Input: part model. Units: mm. Frame: model coordinates. A direction names the side the tool comes from. Coordinates: 2 decimals unless noted, no trailing zeros. Write each loop counter-clockwise with the first axis right and the second up, starting at its lowest first coordinate (ties: lowest second). Pieces come first, ordered by that corner, then holes. Notation, with made-up numbers: (62, -2) - (85, -2) arc R14 cw to (85, 2) - close; hole circle Ø10 at (85.25, -9). An arc over 180 degrees is marked (long way). Use a Markdown table: item, result. Add a question column.
Q1. Mould query, pull axis X, two halves, no side actions, for faces 1 (the face through (-5.568, -4.93, -17.725)), 2 (the face through (4, -10, 11)), 3 (the face through (-8.099, -15.21, 7.597)), 4 (the face through (-20.331, -5, 2)). Classes: released by +X, released by -X, zero draft, split by the parting line, or undercut.
Q2. Set-up query: faces 5 (the face through (-17.32, -19.86, 2.8)), 6 (the face through (9.669, -5, 2)). Return all of +Z, -Z, +X, -X, +Y, -Y with unobstructed straight access to the full face (end or side cutting, diameter ignored); none if empty.
Q3. Section query A-A (z = -2.5). Return the cut outline in (x, y).
Q4. Material intervals for probe 1 along X at (y, z) = (-23.25, 7); probe 2 along Y at (x, z) = (-16.5, 7); probe 3 along X at (y, z) = (-20, 5), sorted ascending. Write a range as from..to.
Q5. Section query D-D (x = -5). Return the cut outline in (y, z), then the cut area to 3 significant figures.
Q6. Section query C-C (y = -8.5). Give the number of separate pieces and of enclosed holes in the cut face, then the cut area to 3 significant figures.
Q7. Section query B-B (x = -1). Return the cut outline in (y, z), then the cut area to 3 significant figures.
Q8. Pin query (flat end, axial travel): P1, Ø6, axis at x = -12, y = -21, coming from the +Z side; P2, Ø1, axis at x = -2.5, z = 6.5, coming from the +Y side; P3, Ø6, axis at y = -25, z = 13.5, coming from the +X side; P4, Ø12, axis at y = -25, z = -5, coming from the +X side. Return the tip coordinate at first contact, or that it passes through.
from build123d import *

# Parameters (mm, degrees)
F0_R     = 12
F1_DEPTH = 10
F2_DEPTH = 30
F3_D     = 12
F3_DEPTH = 50
F3_TIP   = 3.6051637142


with BuildPart() as f1:
    # F0 (on Front) → F1 (new body)
    with BuildSketch(Plane.XZ):
        with BuildLine():
            Line((9.6692045312, -3.2938710881), (9.6692045312, 7.8416576376))
            ThreePointArc((9.6692045312, 7.8416576376), (8.7102254474, 9.9452511488), (7.4580991057, 11.8886826932))
            ThreePointArc((7.4580991057, 11.8886826932), (4.3919227725, 11.9966115161), (4.2839939496, 15.0627878494))
            ThreePointArc((4.2839939496, 15.0627878494), (0.792139449, 17.055965795), (-3.0863641887, 18.1156901498))
            ThreePointArc((-3.0863641887, 18.1156901498), (-5.3307954688, 16.0238932748), (-7.575226749, 18.1156901498))
            ThreePointArc((-7.575226749, 18.1156901498), (-11.4537303867, 17.055965795), (-14.9455848872, 15.0627878494))
            ThreePointArc((-14.9455848872, 15.0627878494), (-14.5367720196, 14.3749809927), (-14.3945039678, 13.5876017738))
            ThreePointArc((-14.3945039678, 13.5876017738), (-15.7108735993, 11.5404490352), (-18.1196900434, 11.8886826932))
            ThreePointArc((-18.1196900434, 11.8886826932), (-19.371816385, 9.9452511488), (-20.3307954688, 7.8416576376))
            Line((-20.3307954688, 7.8416576376), (-20.3307954688, -3.2938710881))
            ThreePointArc((-20.3307954688, -3.2938710881), (-19.371816385, -5.3974645992), (-18.1196900434, -7.3408961436))
            ThreePointArc((-18.1196900434, -7.3408961436), (-15.7108735993, -6.9926624856), (-14.3945039678, -9.0398152242))
            ThreePointArc((-14.3945039678, -9.0398152242), (-14.5367720196, -9.8271944431), (-14.9455848872, -10.5150012998))
            ThreePointArc((-14.9455848872, -10.5150012998), (-11.4537303867, -12.5081792454), (-7.575226749, -13.5679036002))
            ThreePointArc((-7.575226749, -13.5679036002), (-5.3307954688, -11.4761067252), (-3.0863641887, -13.5679036002))
            ThreePointArc((-3.0863641887, -13.5679036002), (0.792139449, -12.5081792454), (4.2839939496, -10.5150012998))
            ThreePointArc((4.2839939496, -10.5150012998), (4.3919227725, -7.4488249665), (7.4580991057, -7.3408961436))
            ThreePointArc((7.4580991057, -7.3408961436), (8.7102254474, -5.3974645992), (9.6692045312, -3.2938710881))
        make_face()
        with Locations((-5.3307954688, 2.2738932748)):
            Circle(F0_R, mode=Mode.SUBTRACT)
        with BuildLine():
            Line((9.6692045312, 7.8416576376), (9.6692045312, 15.5026498301))
            ThreePointArc((9.6692045312, 15.5026498301), (-5.3307954688, 22.2738932748), (-20.3307954688, 15.5026498301))
            Line((-20.3307954688, 15.5026498301), (-20.3307954688, 7.8416576376))
            ThreePointArc((-20.3307954688, 7.8416576376), (-19.371816385, 9.9452511488), (-18.1196900434, 11.8886826932))
            ThreePointArc((-18.1196900434, 11.8886826932), (-18.2354942255, 15.1785920314), (-14.9455848872, 15.0627878494))
            ThreePointArc((-14.9455848872, 15.0627878494), (-11.4537303867, 17.055965795), (-7.575226749, 18.1156901498))
            ThreePointArc((-7.575226749, 18.1156901498), (-5.4099460206, 20.5225006638), (-3.0807954688, 18.2738932748))
            ThreePointArc((-3.0807954688, 18.2738932748), (-3.0821880798, 18.194742723), (-3.0863641887, 18.1156901498))
            ThreePointArc((-3.0863641887, 18.1156901498), (0.792139449, 17.055965795), (4.2839939496, 15.0627878494))
            ThreePointArc((4.2839939496, 15.0627878494), (6.770292249, 15.695333722), (8.2329130301, 13.5876017738))
            ThreePointArc((8.2329130301, 13.5876017738), (8.0300657687, 12.6539714053), (7.4580991057, 11.8886826932))
            ThreePointArc((7.4580991057, 11.8886826932), (8.7102254474, 9.9452511488), (9.6692045312, 7.8416576376))
        make_face()
        with BuildLine():
            ThreePointArc((-20.3307954688, -10.9548632805), (-5.3307954688, -17.7261067252), (9.6692045312, -10.9548632805))
            Line((9.6692045312, -10.9548632805), (9.6692045312, -3.2938710881))
            ThreePointArc((9.6692045312, -3.2938710881), (8.7102254474, -5.3974645992), (7.4580991057, -7.3408961436))
            ThreePointArc((7.4580991057, -7.3408961436), (8.0300657687, -8.1061848557), (8.2329130301, -9.0398152242))
            ThreePointArc((8.2329130301, -9.0398152242), (6.770292249, -11.1475471725), (4.2839939496, -10.5150012998))
            ThreePointArc((4.2839939496, -10.5150012998), (0.792139449, -12.5081792454), (-3.0863641887, -13.5679036002))
            ThreePointArc((-3.0863641887, -13.5679036002), (-3.0821880798, -13.6469561734), (-3.0807954688, -13.7261067252))
            ThreePointArc((-3.0807954688, -13.7261067252), (-5.4099460206, -15.9747141143), (-7.575226749, -13.5679036002))
            ThreePointArc((-7.575226749, -13.5679036002), (-11.4537303867, -12.5081792454), (-14.9455848872, -10.5150012998))
            ThreePointArc((-14.9455848872, -10.5150012998), (-18.2354942255, -10.6308054819), (-18.1196900434, -7.3408961436))
            ThreePointArc((-18.1196900434, -7.3408961436), (-19.371816385, -5.3974645992), (-20.3307954688, -3.2938710881))
            Line((-20.3307954688, -3.2938710881), (-20.3307954688, -10.9548632805))
        make_face()
        with Locations((-5.3307954688, 2.2738932748)):
            Circle(F0_R)
    extrude(amount=F1_DEPTH)

    # F0 (on Front) → F2 (join)
    with BuildSketch(Plane.XZ):
        with Locations((-5.3307954688, 2.2738932748)):
            Circle(F0_R)
    extrude(amount=F2_DEPTH)

    # F3
    with Locations(Plane(origin=(0, 0, 0), x_dir=(1, 0, 0), z_dir=(0, 1, 0))):
        with Locations((-5.3307954688, -2.2738932748)):
            Hole(F3_D / 2, depth=F3_DEPTH)
            with Locations((0, 0, -(F3_DEPTH + F3_TIP / 2))):  # 118° drill point
                Cone(0, F3_D / 2, F3_TIP, mode=Mode.SUBTRACT)


solid = f1.part
Values follow:
| question | item | result |
|---|---|---|
| 1 | face 1 | split by the parting line |
| 1 | face 2 | zero draft |
| 1 | face 3 | undercut |
| 1 | face 4 | released by -X |
| 2 | face 5 | -Y |
| 2 | face 6 | +Z, -Z, +X, +Y, -Y |
| 3 | outline | (-20.33, -10) - (-16.34, -10) - (-16.34, -30) - (-8.97, -30) - (-8.97, 0) - (-20.33, 0) - close; (-1.7, -30) - (5.68, -30) - (5.68, -10) - (9.67, -10) - (9.67, 0) - (-1.7, 0) - close |
| 4 | probe 1 | -16.36..-9.03, -1.63..5.7 |
| 4 | probe 2 | -10..0 |
| 4 | probe 3 | -17.02..-10.68, 0.01..6.36 |
| 5 | outline | (-30, -9.72) - (-10, -9.72) - (-10, -11.5) - (0, -11.5) - (0, -3.72) - (-30, -3.72) - close; (-30, 8.26) - (0, 8.26) - (0, 16.05) - (-10, 16.05) - (-10, 14.27) - (-30, 14.27) - close; (-10, -17.72) - (0, -17.72) - (0, -15.95) - (-10, -15.95) - close; (-10, 20.5) - (0, 20.5) - (0, 22.27) - (-10, 22.27) - close |
| 5 | area | 431 mm2 |
| 6 | separate pieces | 1 |
| 6 | enclosed holes | 7 |
| 6 | area | 867 mm2 |
| 7 | outline | (-30, -8.92) - (-10, -8.92) - (-10, -17.25) - (0, -17.25) - (0, -1.88) - (-30, -1.88) - close; (-30, 6.43) - (0, 6.43) - (0, 21.8) - (-10, 21.8) - (-10, 13.47) - (-30, 13.47) - close |
| 7 | area | 589 mm2 |
| 8 | P1 | z = 13.7 |
| 8 | P2 | through |
| 8 | P3 | x = 3.41 |
| 8 | P4 | x = 6.6 |
